```python
from build123d import *

# Parameters (mm, degrees)
SKETCH1_R           = 5
BOSS_EXTRUDE1_DEPTH = 25
CUT_EXTRUDE1_DEPTH  = 2.05


with BuildPart() as part:
    # Sketch1 → Boss-Extrude1 (new body)
    with BuildSketch(Plane(origin=(0, 0, 0), x_dir=(1, 0, 0), z_dir=(0, 1, 0))):
        with Locations(Location((0, 0, 0), (0, 0, 270))):
            Circle(SKETCH1_R)
    extrude(amount=BOSS_EXTRUDE1_DEPTH)

    # Sketch2 → Cut-Extrude1 (cut, symmetric)
    with BuildSketch(Plane.XY):
        with BuildLine():
            Line((-4, 11.5), (-4, 25))
            Line((-4, 25), (4, 25))
            Line((4, 25), (4, 11.5))
            ThreePointArc((4, 11.5), (0, 7.5), (-4, 11.5))
        make_face()
    extrude(amount=CUT_EXTRUDE1_DEPTH, both=True, mode=Mode.SUBTRACT)


solid = part.part
```
Source: CAD feature listing. Evaluate the final solid. Frame: model axes, mm. A direction names the side the tool comes from. Coordinates: 2 decimals unless noted, no trailing zeros. Order: outer loops, then holes, each group sorted by start corner. A loop starts at its lowest first (then second) coordinate and runs counter-clockwise, first axis right, second up. Notation, with made-up numbers: M 35,-31.5 L 94,-31.5 A24 ccw 94,1.5 Z; hole C 53.5,-34 d6. An arc over 180 degrees is marked long. Write each question's results on one line, items separated by ' | '. Start each with the question number.
1) Section query B-B (x = 0). Return the cut outline in (y, z), plus the area to 3 significant figures.
2) Section query C-C (y = 14.5). Return the cut outline in (x, z).
3) Line query: line 1 (Z direction, x = 3, y = 15.75); line 2 (Z direction, x = 3, y = 6.25); line 3 (X direction, y = 12.5, z = 1.5). Output: solid intervals per line, ascending. Write a range as from..to.
4) Contact query for flat-ended pins moving along their axis: pin 1 Ø1 at (y, z) = (11.5, 3.5) entering from -X; pin 2 Ø1.5 at (y, z) = (10, -2.5) entering from -X; pin 3 Ø1 at (x, z) = (2, 1) entering from +Y. Output: stop coordinate, or through.
5) Section query A-A (z = 0). Return the cut outline in (x, y), plus the area to 3 significant figures.
6) Draft query along Z for faces 3 (the face through (0.1, 25, 2.2)), 4 (the face through (0, 16, 2.05)), 5 (the face through (0.1, 7.5, 0)), 6 (the face through (-4.88, 12.32, -1.08)). Return one class per face: released by +Z, released by -Z, zero draft, split by the parting line, or undercut.
7) Section query D-D (x = 4.25). Return the cut outline in (y, z), plus the area to 3 significant figures.
8) Access query for faces 1 (the face through (0, 16, -2.05)), 2 (the face through (0, 0, 0)). Directions: +Z, -Z, +X, -X, +Y, -Y. A direction counts if a zero-diameter tool reaches every point of the face in a straight line with its end or side. Return the directions, or none.
Answers:
1) outline: M 0,-5 L 25,-5 L 25,-2.05 L 7.5,-2.05 L 7.5,2.05 L 25,2.05 L 25,5 L 0,5 Z | area: 178 mm^2
2) outline: C 0,0 d10; hole M -4,-2.05 L 4,-2.05 L 4,2.05 L -4,2.05 Z
3) line 1: z = -4..-2.05, 2.05..4 | line 2: z = -4..4 | line 3: x = -4.77..-4, 4..4.77
4) pin 1: stops at x = -4 | pin 2: stops at x = -4.68 | pin 3: stops at y = 8.38
5) outline: M -5,0 L 5,0 L 5,25 L 4,25 L 4,11.5 A4 cw -4,11.5 L -4,25 L -5,25 Z | area: 117 mm^2
6) face 3: zero draft | face 4: undercut | face 5: undercut | face 6: split by the parting line
7) outline: M 0,-2.63 L 25,-2.63 L 25,2.63 L 0,2.63 Z | area: 132 mm^2
8) face 1: +Y | face 2: +Z, -Z, +X, -X, -Y
